from build123d import *

# Parameters (mm, degrees)
F1_ANGLE  = 270
F5_DEPTH  = 1
F7_DEPTH  = 1
F8_R      = 2.3999784267
F9_DEPTH  = 0.5
F10_R     = 2.2479266401
F11_DEPTH = 0.5
F12_R     = 2.219715214
F13_DEPTH = 0.5
F14_R     = 2.225517588
F15_DEPTH = 0.5
F21_DEPTH = 1


# Not quite as in the source:
# - the program builds the solid bodies; features that only make, move or delete a surface that nothing else refers to are left out


with BuildPart() as f1:
    # F0 (on Right) → F1 (revolve)
    with BuildSketch(Plane.YZ):
        with BuildLine():
            Line((30.0334315861, 0), (-29.9665684139, 0))
            ThreePointArc((-29.9665684139, 0), (0.0334315861, -30), (30.0334315861, 0))
        make_face()
    revolve(axis=Axis((0, 0.0334315861, 0), (0, 1, 0)), revolution_arc=F1_ANGLE)

    # F2 (on face) → F3 (revolve)
    with BuildSketch(Plane.YZ):
        with BuildLine():
            Line((0, -13.9990693861), (0, 0))
            Line((0, 0), (-0.1614197102, 0))
            ThreePointArc((-0.1614197102, 0), (-7.0802445482, -7.0802445482), (0, -13.9990693861))
        make_face()
        with BuildLine():
            Line((0, -13.9990693861), (0, 0))
            ThreePointArc((0, 0), (-7.0807098551, -6.9995346931), (0, -13.9990693861))
        make_face()
    revolve(axis=Axis((0, 0, -6.9995346931), (0, 0, -1)))

    # F4 (on Right) → F5 (join)
    with BuildSketch(Plane.YZ):
        with BuildLine():
            add(Edge.make_bspline(
                [(17.0095134526, -15.6440958381), (20.8283990638, -15.6440958381), (18.9189562582, -6.4476504922), (17.0095134526, 2.7487948537), (15.1000706471, -6.4476504922), (13.1906278415, -15.6440958381), (17.0095134526, -15.6440958381)],
                knots=[0, 0, 0, 2.0943951024, 2.0943951024, 4.1887902048, 4.1887902048, 6.2831853072, 6.2831853072, 6.2831853072], degree=2, weights=[1, 0.5, 1, 0.5, 1, 0.5, 1]))
        make_face()
    extrude(amount=F5_DEPTH)

    # F6 (on Right) → F7 (join)
    with BuildSketch(Plane.YZ):
        with BuildLine():
            add(Edge.make_bspline(
                [(-14.6672427654, -18.0654972792), (-11.4328069704, -15.6641534543), (-19.325768114, -8.4118548322), (-27.2187292576, -1.15955621), (-22.560203909, -10.8131986571), (-17.9016785604, -20.4668411041), (-14.6672427654, -18.0654972792)],
                knots=[0, 0, 0, 2.0943951024, 2.0943951024, 4.1887902048, 4.1887902048, 6.2831853072, 6.2831853072, 6.2831853072], degree=2, weights=[1, 0.5, 1, 0.5, 1, 0.5, 1]))
        make_face()
    extrude(amount=F7_DEPTH)

    # F8 (on face) → F9 (join)
    with BuildSketch(Plane.YZ):
        with Locations((-6.5264105797, -22.420451045)):
            Circle(F8_R)
    extrude(amount=F9_DEPTH)

    # F10 (on face) → F11 (join)
    with BuildSketch(Plane(origin=(0, 0, 0), x_dir=(1, 0, 0), z_dir=(0, 0, -1))):
        with Locations((5.2993446589, -22.5904844701)):
            Circle(F10_R)
    extrude(amount=F11_DEPTH)

    # F12 (on face) → F13 (join)
    with BuildSketch(Plane(origin=(0, 0, 0), x_dir=(1, 0, 0), z_dir=(0, 0, -1))):
        with Locations((25.2750441432, 3.729365766)):
            Circle(F12_R)
    extrude(amount=F13_DEPTH)

    # F14 (on face) → F15 (join)
    with BuildSketch(Plane(origin=(0, 0, 0), x_dir=(1, 0, 0), z_dir=(0, 0, -1))):
        with Locations((11.6383302957, 21.1235657334)):
            Circle(F14_R)
    extrude(amount=F15_DEPTH)

    # F20 (on face) → F21 (join)
    with BuildSketch(Plane(origin=(0, 0, 0), x_dir=(1, 0, 0), z_dir=(0, 0, -1))):
        with BuildLine():
            add(Edge.make_bspline(
                [(7.3144584894, -10.2911405265), (10.5177671604, -12.9900925853), (13.6132754829, -6.0656891234), (16.7087838054, 0.8587143384), (10.4099668119, -3.3667370647), (4.1111498184, -7.5921884678), (7.3144584894, -10.2911405265)],
                knots=[0, 0, 0, 2.0943951024, 2.0943951024, 4.1887902048, 4.1887902048, 6.2831853072, 6.2831853072, 6.2831853072], degree=2, weights=[1, 0.5, 1, 0.5, 1, 0.5, 1]))
        make_face()
    extrude(amount=F21_DEPTH)


solid = f1.part
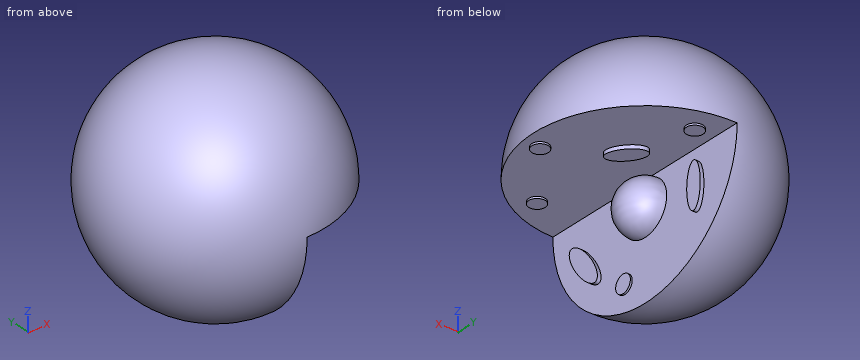
Geometry: final body of the model. Coordinates: model frame, mm. Coordinates: 2 decimals unless noted, no trailing zeros. Order: outer loops, then holes, each group sorted by start corner. A loop starts at its lowest first (then second) coordinate and runs counter-clockwise, first axis right, second up.
(1) First-contact query: pin 1 (5 mm diameter, centred on y = 16.5, z = -10, fed in from +X); pin 2 (2 mm diameter, centred on y = -19.5, z = -17.5, fed in from -X); pin 3 (2 mm diameter, centred on x = 4.5, y = 23, fed in from -Z). Flat tips, straight axial feed; report the tip coordinate or a pass-through.
(2) Section query A-A (z = -21). Return the cut outline in (x, y), plus the area to 3 significant figures.
(3) Section query D-D (x = -24.5). Return the cut outline in (y, z).
(4) Material intervals for probe 1 along Y at (x, z) = (-17, -15.5); probe 2 along X at (y, z) = (-18, -9); probe 3 along Z at (x, y) = (-6.5, 8.5), sorted ascending.
(5) Section query C-C (z = 19). Return the cut outline in (x, y), plus the area to 3 significant figures.
Solution:
1. pin 1: stops at x = 1
1. pin 2: stops at x = -16.24
1. pin 3: stops at z = -0.5
2. outline: (0, -21.39) - (0, -8.46) - (0.5, -8.46) - (0.5, -4.59) - (0, -4.59) - (0, 21.46) arc R21.42 ccw to start
2. area: 723 mm2
3. outline: circle Ø34.63 at (0.03, 0)
4. probe 1: y = -19.22 to 19.29
4. probe 2: x = -22.22 to 0
4. probe 3: z = -28.04 to 28.04
5. outline: circle Ø46.43 at (0, 0.03)
5. area: 1,690 mm2
